Autodesk Inventor part; units mm, degrees
ref_plane "YZ Plane" through (0, 0, 0) normal (1, 0, 0) x (0, 1, 0)
ref_plane "XZ Plane" through (0, 0, 0) normal (0, 1, 0) x (-1, 0, 0)
ref_plane "XY Plane" through (0, 0, 0) normal (0, 0, 1) x (1, 0, 0)
sketch "Sketch1" plane through (0, 0, 0) normal (0, 0, 1) x (1, 0, 0)
  line L0 (-48.5, 33) -> (48.5, 33)
  line L1 (48.5, 33) -> (48.5, -33)
  line L2 (48.5, -33) -> (-48.5, -33)
  line L3 (-48.5, -33) -> (-48.5, 33)
  point P0 (0, 0)
  point P1 (0, 33)
  point P2 (-48.5, 0)
  dimension "d0" = 97
  dimension "d1" = 66
extrude "Extrusion1" add sketch "Sketch1" along normal blind 8
sketch "Sketch4" plane through (0, 0, 8) normal (0, 0, 1) x (1, 0, 0)
  line L0 (-48.5, 33) -> (-48.5, -33)
  line L1 (-48.5, -33) -> (48.5, -33)
  line L2 (48.5, 33) -> (-48.5, 33)
  point P0 (0, 0)
  point P1 (-38.5, -29)
  point P2 (-38.5, 29)
  dimension "d19" = 10
  dimension "d20" = 4
  dimension "d21" = 4
hole "Hole1" at (-38.5, -29, 8) at (-38.5, 29, 8) direction (0, 0, -1) diameter 4.5 end through all
pattern_linear "Rectangular Pattern1" count 2 spacing 50 along (1, 0, 0) of "Hole1"
properties part number "0005-10-009"
Here's how the part is built. I have some questions about the finished solid (model axes, mm). Coordinates: 2 decimals unless noted, no trailing zeros. Write each loop counter-clockwise with the first axis right and the second up, starting at its lowest first coordinate (ties: lowest second). Pieces come first, ordered by that corner, then holes. Notation, with made-up numbers: M 36,-26 L 50,-26 A25 cw 50,10 Z; hole C 53,46 d3. An arc over 180 degrees is marked long. Answer as CSV lines item,"result". Start each with the question number.
Q1. Will this pin go through, and if not, where does the flat tip stop? pin 1 Ø6 at (x, y) = (-21.5, -22.5) entering from -Z.
Q2. I need wall thicknesses on probe 1 along X at (y, z) = (-29, 5); probe 2 along Y at (x, z) = (-38.5, 2); probe 3 along Y at (x, z) = (-36.5, 7). Which ranges of each line are inside material? Lowest first, please. Write a range as [from, to].
Q3. Suppose I cut it at A-A, the plane y = 29. List the corners of the cut face in (x, z) for me.
Q4. If we mould it in two halves opening along X, with no side actions, what happens to faces 1 (the flat face through (-1, 0, 0)), 2 (the cylindrical face through (-40.397, 27.79, 3.944)), 3 (the flat face through (48.5, 0, 4))? For each: pulls with the +X half, pulls with the -X half, needs draft (parallel to the pull), parting line crosses it, or undercut.
Q5. Suppose I cut it at B-B, the plane x = 11.5. List the corners of the cut face in (y, z) for me, then the cut area to 3 significant figures.
Entries:
1,pin 1,"stops at z = 0"
2,probe 1,"x = [-48.5, -40.75], [-36.25, 9.25], [13.75, 48.5]"
2,probe 2,"y = [-33, -31.25], [-26.75, 26.75], [31.25, 33]"
2,probe 3,"y = [-33, -30.03], [-27.97, 27.97], [30.03, 33]"
3,outline,"M -48.5,0 L -40.75,0 L -40.75,8 L -48.5,8 Z; M -36.25,0 L 9.25,0 L 9.25,8 L -36.25,8 Z; M 13.75,0 L 48.5,0 L 48.5,8 L 13.75,8 Z"
4,face 1,"needs draft"
4,face 2,"undercut"
4,face 3,"pulls with the +X half"
5,outline,"M -33,0 L -31.25,0 L -31.25,8 L -33,8 Z; M -26.75,0 L 26.75,0 L 26.75,8 L -26.75,8 Z; M 31.25,0 L 33,0 L 33,8 L 31.25,8 Z"
5,area,"456 mm²"
